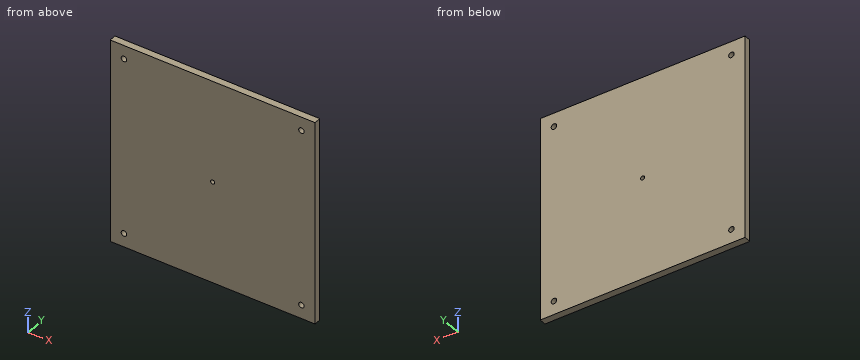
Autodesk Inventor part; units mm, degrees
ref_plane "YZ Plane" through (0, 0, 0) normal (1, 0, 0) x (0, 1, 0)
ref_plane "XZ Plane" through (0, 0, 0) normal (0, 1, 0) x (-1, 0, 0)
ref_plane "XY Plane" through (0, 0, 0) normal (0, 0, 1) x (1, 0, 0)
sketch "Sketch1" plane through (0, 0, 0) normal (0, 1, 0) x (-1, 0, 0)
  line L0 (0, 0) -> (300, 0)
  line L1 (300, 0) -> (300, -300)
  line L2 (300, -300) -> (0, -300)
  line L3 (0, -300) -> (0, 0)
  dimension "d0" = 300
  dimension "d1" = 300
extrude "Extrusion1" add sketch "Sketch1" along normal blind 10
sketch "Sketch2" plane through (0, 10, 0) normal (0, 1, 0) x (1, 0, 0)
  line L0 (-300, 0) -> (0, 0)
  line L1 (0, 0) -> (0, 300)
  point P0 (-20, 20)
  point P1 (-20, 280)
  point P2 (-280, 20)
  point P3 (-280, 280)
  dimension "d4" = 20
  dimension "d5" = 20
  dimension "d8" = 260
  dimension "d11" = 260
hole "Hole1" at (-20, 10, -20) at (-20, 10, -280) at (-280, 10, -20) at (-280, 10, -280) direction (0, -1, 0) diameter 8 end through all
sketch "Sketch3" plane through (0, 10, 0) normal (0, 1, 0) x (1, 0, 0)
  line L0 (-300, 300) -> (-300, 0)
  line L1 (0, 300) -> (-300, 300)
  point P0 (0, 0)
  point P1 (-150, 150)
  dimension "d21" = 150
  dimension "d22" = 150
hole "Hole2" at (-150, 10, -150) direction (0, -1, 0) diameter 6 end through all
properties part number "Plate"
Build history of the part. All positions in model axes, mm. Coordinates: 2 decimals unless noted, no trailing zeros. Order: outer loops, then holes, each group sorted by start corner. A loop starts at its lowest first (then second) coordinate and runs counter-clockwise, first axis right, second up. Notation, with made-up numbers: (7.5, -12) -> (38.5, -12) arc R22 cw to (38.5, 14) -> close; hole circle Ø2 at (43.5, -16). An arc over 180 degrees is marked (long way). Answer in a Markdown table with one row per item. Add a question column.
Q1. Band-saw the part on A-A, the plane x = -20. List the corners of the cut face in (y, z).
Q2. Drop a flat-ended pin along its axis: pin 1 (6 mm diameter, centred on x = -85.5, y = 1.5, fed in from +Z). Give the stop position or say it passes through.
Q3. Band-saw the part on B-B, the plane z = -20. List the corners of the cut face in (x, y), then the cut area to 3 significant figures.
Q4. Wall check: line 1 along Z through (x, y) = (-280, 5); line 2 along Z through (x, y) = (-150, 6.25). Give the ranges that are in metal, low to high. Write a range as [from, to].
Answers follow:
| question | item | result |
|---|---|---|
| 1 | outline | (0, -300) -> (10, -300) -> (10, -284) -> (0, -284) -> close; (0, -276) -> (10, -276) -> (10, -24) -> (0, -24) -> close; (0, -16) -> (10, -16) -> (10, 0) -> (0, 0) -> close |
| 2 | pin 1 | z = 0 |
| 3 | outline | (-300, 0) -> (-284, 0) -> (-284, 10) -> (-300, 10) -> close; (-276, 0) -> (-24, 0) -> (-24, 10) -> (-276, 10) -> close; (-16, 0) -> (0, 0) -> (0, 10) -> (-16, 10) -> close |
| 3 | area | 2,840 mm^2 |
| 4 | line 1 | [-300, -284], [-276, -24], [-16, 0] |
| 4 | line 2 | [-300, -153], [-147, 0] |
